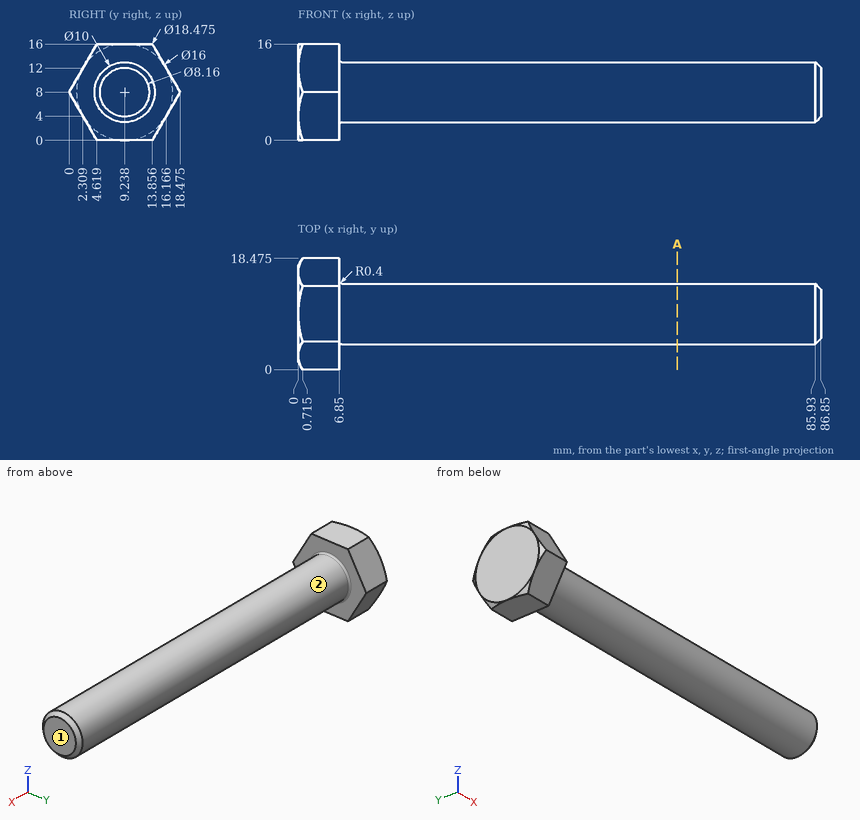
Can you work these out from the drawing? Everything is in mm from the part's minimum corner. A direction names the side the tool comes from. Round coordinates to 2 decimals unless told otherwise and drop trailing zeros. Loops run counter-clockwise (first coordinate to the right, second up) from the corner with the lowest first, then second, coordinate; pieces in that order, holes last. Notation, with made-up numbers: (47.25, -10) -> (72.25, -10) arc R11 ccw to (72.25, 8) -> close; hole circle Ø9 at (29, 48.25). An arc over 180 degrees is marked (long way). Put each result on its own line as item: value.
Q1. I want a section at A-A on x = 63. Write out the boundary of the cut face in (y, z).
Checks:
outline: circle Ø10 at (9.24, 8)
Q2. Which directions (+Z, -Z, +X, -X, +Y, -Y) give clear straight access to the entire face, cutting with the end or side of a thin tool? Please do the marked faces 1 and 2.
Checks:
face 1: +Z, -Z, +X, +Y, -Y
face 2: +X
Q3. Please list where these lines run through material, in increasing order: line 1 (X direction, y = 4.25, z = 5.25); line 2 (Z direction, x = 62, y = 9) (1 decimal); line 3 (Z direction, x = 78.5, y = 11.25). Write a range as from..to.
Checks:
line 1: 0..6.85
line 2: 3..13
line 3: 3.42..12.58
Q4. For pin 1 Ø2 at (x, z) = (49, 9) entering from -Y; pin 2 Ø1.5 at (x, y) = (42, 7) entering from -Z; pin 3 Ø4 at (x, z) = (59.5, 2) entering from +Y; pin 4 Ø1 at (x, y) = (23, 16) entering from +Z, each with a flat end and sliding along its axis, tell me the tip position at first contact or that it passes through.
Checks:
pin 1: y = 4.24
pin 2: z = 3.23
pin 3: y = 12.24
pin 4: through
